```python
from build123d import *

# Parameters (mm, degrees)
F1_DEPTH  = 25.4
F2_R      = 13.276000262
F2_R_2    = 13.2682995005
F3_DEPTH  = 25.401
F4_W      = 93.4033617377
F4_H      = 26.7108418047
F5_DEPTH  = 38.1
F7_DEPTH  = 38.7764468004
F8_W      = 13.8678809612
F8_H      = 13.3554209024
F10_W     = 13.8678809612
F10_H     = 13.3554209024
F12_R     = 7.2961066279
F13_DEPTH = 148.2995960076


with BuildPart() as f1:
    # F0 (on Top) → F1 (new body)
    with BuildSketch(Plane.XY):
        with BuildLine():
            ThreePointArc((-76.1768892407, 25.420025898), (-58.2022165503, 17.9746726904), (-50.7568633427, 0))
            ThreePointArc((-50.7568633427, 0), (-58.0842609925, -17.8559379403), (-75.8421658524, -25.4178220332))
            Line((-75.8421658524, -25.4178220332), (75.9601819019, -25.4294734106))
            ThreePointArc((75.9601819019, -25.4294734106), (50.5350089445, -0.3456126871), (75.2690210938, 25.420025898))
            Line((75.2690210938, 25.420025898), (-76.1768892407, 25.420025898))
        make_face()
        with BuildLine():
            ThreePointArc((-75.8421658524, -25.4178220332), (-58.0842609925, -17.8559379403), (-50.7568633427, 0))
            ThreePointArc((-50.7568633427, 0), (-58.2022165503, 17.9746726904), (-76.1768892407, 25.420025898))
            ThreePointArc((-76.1768892407, 25.420025898), (-101.5963512458, 0.1693163576), (-76.5155144441, -25.4177703512))
            Line((-76.5155144441, -25.4177703512), (-75.8421658524, -25.4178220332))
        make_face()
        with BuildLine():
            Line((76.6552463174, 25.420025898), (75.2690210938, 25.420025898))
            ThreePointArc((75.2690210938, 25.420025898), (50.5350089445, -0.3456126871), (75.9601819019, -25.4294734106))
            ThreePointArc((75.9601819019, -25.4294734106), (93.9427967691, -17.9820431972), (101.3916071911, 0))
            ThreePointArc((101.3916071911, 0), (94.186891736, 17.7346078751), (76.6552463174, 25.420025898))
        make_face()
    extrude(amount=-F1_DEPTH)

    # F2 (on face) → F3 (cut, through all)
    with BuildSketch(Plane.XY):
        with Locations((-76.5155144441, 0)):
            Circle(F2_R)
        with Locations((76.1081134062, 0)):
            Circle(F2_R_2)
    extrude(amount=-F3_DEPTH, mode=Mode.SUBTRACT)

    # F4 (on face) → F5 (join)
    with BuildSketch(Plane.XY):
        Rectangle(F4_W, F4_H)
    extrude(amount=F5_DEPTH)

    # F6 (on face) → F7 (cut, through all)
    with BuildSketch(Plane.XZ.offset(13.3554209024)):
        with BuildLine():
            ThreePointArc((-32.8337999076, 38.1), (0, 5.2662000924), (32.8337999076, 38.1))
            Line((32.8337999076, 38.1), (-32.8337999076, 38.1))
        make_face()
        with BuildLine():
            Line((-32.8337999076, 38.1), (32.8337999076, 38.1))
            ThreePointArc((32.8337999076, 38.1), (0, 70.9337999076), (-32.8337999076, 38.1))
        make_face()
    extrude(amount=-F7_DEPTH, mode=Mode.SUBTRACT)

    # F8 (on face) → F9 (revolve)
    with BuildSketch(Plane.XY.offset(38.1)):
        with Locations((39.7677403882, 6.6777104512)):
            Rectangle(F8_W, F8_H)
    revolve(axis=Axis((39.7677403882, 0, 38.1), (-1, 0, 0)))

    # F10 (on face) → F11 (revolve)
    with BuildSketch(Plane.XY.offset(38.1)):
        with Locations((-39.7677403882, 6.6777104512)):
            Rectangle(F10_W, F10_H)
    revolve(axis=Axis((-39.7677403882, 0, 38.1), (-1, 0, 0)))

    # F12 (on face) → F13 (cut, through all)
    with BuildSketch(Plane.YZ.offset(46.7016808689)):
        with Locations((0, 38.1)):
            Circle(F12_R)
    extrude(amount=-F13_DEPTH, mode=Mode.SUBTRACT)


solid = f1.part
```
Input: part model. Units: mm. Frame: model coordinates. A direction names the side the tool comes from. Give positions to 0.01 mm unless a question says otherwise; leave off trailing zeros. Loops run counter-clockwise (first coordinate to the right, second up) from the corner with the lowest first, then second, coordinate; pieces in that order, holes last. Notation, with made-up numbers: M 25.5,49 L 46.5,49 A26 cw 46.5,65 Z; hole C -30.75,-26 d2. An arc over 180 degrees is marked long. Answer as CSV lines item,"result". Start each with the question number.
1. Pin query (flat end, axial travel): P1, Ø4, axis at y = 20, z = -7, coming from the -X side; P2, Ø14.5, axis at y = 4, z = 46.5, coming from the -X side; P3, Ø8, axis at y = 3, z = 38, coming from the +X side; P4, Ø6, axis at x = 33.5, z = 39.5, coming from the -Y side. Return the tip coordinate at first contact, or that it passes through.
2. Pull-direction query (Z, two-part tool) for faces 5 (the face through (39.865, -0.294, 51.452)), 6 (the face through (46.702, 0, 20)), 7 (the face through (-39.254, -1.582, 30.977)); classes: released by +Z, released by -Z, zero draft, split by the parting line, or undercut.
3. Section A-A on y = 0. Return loops of the section in (x, z).
4. Section C-C on x = 73. Return loops of the section in (y, z).
5. Section D-D on y = -11. Return loops of the section in (x, z), plus the area to 3 significant figures.
6. Reachability of faces 1 (the face through (-46.702, 0, 20)), 2 (the face through (-1, 13.355, 2)), 3 (the face through (32.834, 0, 46)), 4 (the face through (-1, -13.355, 2)) from +Z, -Z, +X, -X, +Y, -Y: full face, straight path, thin tool, end or side. Return the list, or none.
7. Line query: L1, parallel to Z at x = -42.25, y = 0; L2, parallel to X at y = -8.5, z = 37; L3, parallel to Y at x = 40.5, z = 38.1. Output: solid intervals per line, ascending.
8. Section B-B on z = 41. Return loops of the section in (x, y), plus the area to 3 significant figures.
Computed values:
1,P1,"stops at x = -94.13"
1,P2,"stops at x = -46.7"
1,P3,"passes through"
1,P4,"stops at y = -13.36"
2,face 5,"released by +Z"
2,face 6,"zero draft"
2,face 7,"undercut"
3,outline,"M -101.6,-25.4 L -89.79,-25.4 L -89.79,0 L -101.6,0 Z; M -63.24,-25.4 L 62.84,-25.4 L 62.84,0 L 46.7,0 L 46.7,30.8 L 32.01,30.8 A32.83 cw -32.01,30.8 L -46.7,30.8 L -46.7,0 L -63.24,0 Z; M -46.7,45.4 L -32.83,45.4 L -32.83,51.46 L -46.7,51.46 Z; M 32.83,45.4 L 46.7,45.4 L 46.7,51.46 L 32.83,51.46 Z; M 89.38,-25.4 L 101.39,-25.4 L 101.39,0 L 89.38,0 Z"
4,outline,"M -25.43,-25.4 L -12.9,-25.4 L -12.9,0 L -25.43,0 Z; M 12.9,-25.4 L 25.42,-25.4 L 25.42,0 L 12.9,0 Z"
5,outline,"M -99.09,-25.4 L -83.95,-25.4 L -83.95,0 L -99.09,0 Z; M -69.08,-25.4 L 68.69,-25.4 L 68.69,0 L 46.7,0 L 46.7,45.67 L 32.83,45.67 L 32.83,38.1 A32.83 cw -32.83,38.1 L -32.83,45.67 L -46.7,45.67 L -46.7,0 L -69.08,0 Z; M 83.53,-25.4 L 98.89,-25.4 L 98.89,0 L 83.53,0 Z"
5,area,"6,350 mm²"
6,face 1,"+Z, -X, +Y, -Y"
6,face 2,"+Z, +X, -X, +Y"
6,face 3,"+Z, +Y, -Y"
6,face 4,"+Z, +X, -X, -Y"
7,L1,"z = -25.4 to 30.8, 45.4 to 51.46"
7,L2,"x = -46.7 to -32.82, 32.82 to 46.7"
7,L3,"y = -13.36 to -7.3, 7.3 to 13.36"
8,outline,"M -46.7,-13.04 L -32.83,-13.04 L -32.83,-6.7 L -46.7,-6.7 Z; M -46.7,6.7 L -32.83,6.7 L -32.83,13.04 L -46.7,13.04 Z; M 32.83,-13.04 L 46.7,-13.04 L 46.7,-6.7 L 32.83,-6.7 Z; M 32.83,6.7 L 46.7,6.7 L 46.7,13.04 L 32.83,13.04 Z"
8,area,"352 mm²"
